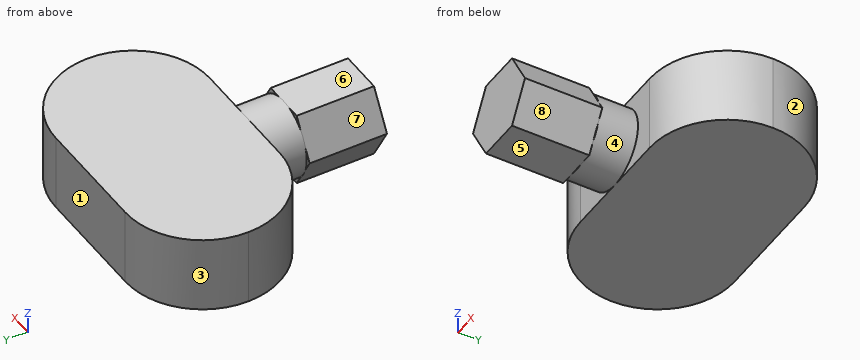
from build123d import *

# Parameters (mm, degrees)
BOSS_EXTRUDE1_DEPTH = 4
SKETCH3_R           = 1.991858429
BOSS_EXTRUDE3_DEPTH = 2
SKETCH2_W           = 14
SKETCH2_H           = 4
BOSS_EXTRUDE2_DEPTH = 8
FILLET1_R           = 4


with BuildPart() as part:
    # Sketch1 → Boss-Extrude1 (new body)
    with BuildSketch(Plane(origin=(0, 0, 0), x_dir=(1, 0, 0), z_dir=(0, 1, 0))):
        Polygon((1.125, 1.948557159), (-1.125, 1.948557159), (-2.25, 0), (-1.125, -1.948557159), (1.125, -1.948557159), (2.25, 0), align=None)
    extrude(amount=BOSS_EXTRUDE1_DEPTH)

    # Sketch3 → Boss-Extrude3 (add)
    with BuildSketch(Plane(origin=(0, 4, 0), x_dir=(1, 0, 0), z_dir=(0, 1, 0))):
        with Locations(Location((0, 0, 0), (0, 0, 78.031254445))):
            Circle(SKETCH3_R)
    extrude(amount=BOSS_EXTRUDE3_DEPTH)

    # Sketch2 → Boss-Extrude2 (add)
    with BuildSketch(Plane(origin=(0, 6, 0), x_dir=(1, 0, 0), z_dir=(0, 1, 0))):
        Rectangle(SKETCH2_W, SKETCH2_H)
    extrude(amount=BOSS_EXTRUDE2_DEPTH)

    # Fillet1
    fillet1_edges = [part.edges().sort_by_distance(p)[0] for p in [
        (7, 6, 0),
        (7, 14, 0),
        (-7, 6, 0),
        (-7, 14, 0),
    ]]
    fillet(fillet1_edges, radius=FILLET1_R - 0.0001)  # a hair under: the kernel refuses the full size


solid = part.part
Check sheet for the modelled part. Datum: model origin and axes. Units: mm. Face numbers are marked on the shaded views. A direction names the side the tool comes from. Round coordinates to 2 decimals unless told otherwise and drop trailing zeros. Loops run counter-clockwise (first coordinate to the right, second up) from the corner with the lowest first, then second, coordinate; pieces in that order, holes last. Notation, with made-up numbers: (-24, -6.75) - (-19, -6.75) arc R18 cw to (-19, 0.25) - close; hole circle Ø8 at (6.25, 86). An arc over 180 degrees is marked (long way). Answer as CSV lines item,"result". Start each with the question number.
Item 1: Depth check by flat-ended pin: P1, Ø1.8, axis at x = 0, y = 2.5, coming from the -Z side; P2, Ø1.8, axis at x = 0.5, y = 2, coming from the +Z side. Enter the tip coordinate at first touch or a pass-through.
Item 2: Section check B-B (x = -0.75). Record the boundary of the cut face in (y, z).
Item 3: Section check C-C (y = 7). Record the boundary of the cut face in (x, z), and give its area (3 significant figures).
Item 4: Set-up check for the marked faces 4, 5, 6, 7 and 8: record each of +Z, -Z, +X, -X, +Y, -Y from which the full face is reachable in a straight line by a thin tool's end or side.
Item 5: Scan lines: line 1 (Z direction, x = 0.25, y = 1.5); line 2 (X direction, y = 13, z = 0.8); line 3 (X direction, y = 1.5, z = 1.65). Record each from-to range of solid material in increasing order. Write a range as [from, to].
Item 6: Release check for a two-part mould opening along X. For the marked faces 1, 2 and 3 record: +X half, -X half, draft (parallel to the pull), parting line (faces both ways), or undercut.
Report:
1,P1,"stops at z = -1.95"
1,P2,"stops at z = 1.95"
2,outline,"(0, -1.95) - (4, -1.95) - (4, -1.85) - (6, -1.85) - (6, -2) - (14, -2) - (14, 2) - (6, 2) - (6, 1.85) - (4, 1.85) - (4, 1.95) - (0, 1.95) - close"
3,outline,"(-5.65, -2) - (5.65, -2) - (5.65, 2) - (-5.65, 2) - close"
3,area,"45.2 mm2"
4,face 4,"none"
4,face 5,"-Z, +X, -X, -Y"
4,face 6,"+Z, +X, -X, -Y"
4,face 7,"+Z, -X, -Y"
4,face 8,"-Z, +X, -Y"
5,line 1,"z = [-1.95, 1.95]"
5,line 2,"x = [-5.65, 5.65]"
5,line 3,"x = [-1.3, 1.3]"
6,face 1,"draft"
6,face 2,"+X half"
6,face 3,"-X half"
